The listing builds one solid part. Answer for the finished solid, in the listing's coordinates (mm). Give positions to 0.01 mm unless a question says otherwise; leave off trailing zeros. Loops run counter-clockwise (first coordinate to the right, second up) from the corner with the lowest first, then second, coordinate; pieces in that order, holes last. Notation, with made-up numbers: (81, -39.5) -> (89, -39.5) arc R5 cw to (89, -33.5) -> close; hole circle Ø1 at (-35.75, 65.25). An arc over 180 degrees is marked (long way). One line per question, with ' | ' between items. Start each with the question number.
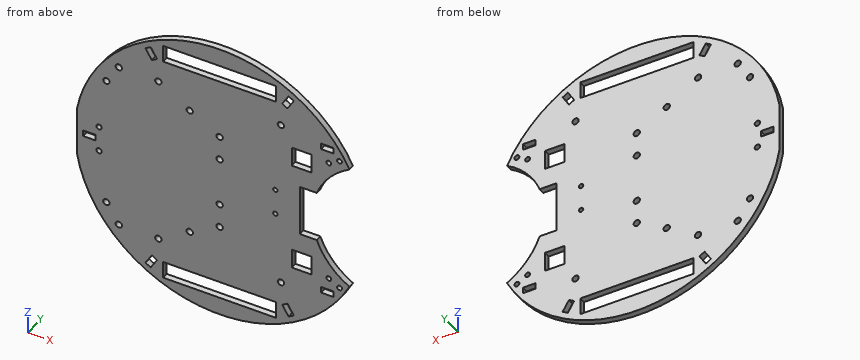
from build123d import *

# Parameters (mm, degrees)
SKETCH1_R           = 1.397
SKETCH1_R_2         = 1.651
SKETCH1_R_3         = 1.143
SKETCH1_R_4         = 1.27
SKETCH1_W           = 58.544107304
SKETCH1_H           = 8.89
SKETCH1_W_2         = 6.35
SKETCH1_H_2         = 3.175
SKETCH1_W_3         = 10.16
SKETCH1_H_3         = 10.16
BOSS_EXTRUDE1_DEPTH = 3.175


with BuildPart() as part:
    # Sketch1 → Boss-Extrude1 (new body)
    with BuildSketch(Plane(origin=(0, 0, 0), x_dir=(1, 0, 0), z_dir=(0, 1, 0))):
        with BuildLine():
            Line((50.342102347, 13.335), (41.582265908, 13.335))
            Line((41.582265908, 13.335), (41.582265908, -13.335))
            Line((41.582265908, -13.335), (50.342102347, -13.335))
            ThreePointArc((50.342102347, -13.335), (52.41895011, -17.937530518), (55.086193863, -22.225))
            ThreePointArc((55.086193863, -22.225), (60.584216496, -28.355013333), (67.270928268, -33.160552015))
            ThreePointArc((67.270928268, -33.160552015), (-10.756431789, -74.224653419), (-73.916912814, -12.7))
            Line((-73.916912814, -12.7), (-73.916912814, 12.7))
            ThreePointArc((-73.916912814, 12.7), (-10.756431789, 74.224653419), (67.270928268, 33.160552015))
            ThreePointArc((67.270928268, 33.160552015), (57.058059725, 24.74076345), (50.342102347, 13.335))
        make_face()
        with Locations(Location((-62.486912814, 6.731, 0), (0, 0, 270))):
            Circle(SKETCH1_R, mode=Mode.SUBTRACT)
        with Locations(Location((-62.486912814, -6.731, 0), (0, 0, 270))):
            Circle(SKETCH1_R, mode=Mode.SUBTRACT)
        with Locations(Location((-31.75, -44.507461806, 0), (0, 0, 270))):
            Circle(SKETCH1_R_2, mode=Mode.SUBTRACT)
        with Locations(Location((31.75, -44.507461806, 0), (0, 0, 270))):
            Circle(SKETCH1_R_2, mode=Mode.SUBTRACT)
        with Locations(Location((31.75, 44.507461806, 0), (0, 0, 90))):
            Circle(SKETCH1_R_2, mode=Mode.SUBTRACT)
        with Locations(Location((0, -12.757461806, 0), (0, 0, 270))):
            Circle(SKETCH1_R_2, mode=Mode.SUBTRACT)
        with Locations(Location((-31.75, 44.507461806, 0), (0, 0, 90))):
            Circle(SKETCH1_R_2, mode=Mode.SUBTRACT)
        with Locations(Location((0, 12.757461806, 0), (0, 0, 90))):
            Circle(SKETCH1_R_2, mode=Mode.SUBTRACT)
        with Locations(Location((28.882265908, 6.731, 0), (0, 0, 270))):
            Circle(SKETCH1_R_3, mode=Mode.SUBTRACT)
        with Locations(Location((-58.676912814, 34.29, 0), (0, 0, 270))):
            Circle(SKETCH1_R_2, mode=Mode.SUBTRACT)
        with Locations(Location((62.141053559, -35.830642926, 0), (0, 0, 270))):
            Circle(SKETCH1_R_4, mode=Mode.SUBTRACT)
        with Locations(Location((56.570777105, -32.679132142, 0), (0, 0, 270))):
            Circle(SKETCH1_R_4, mode=Mode.SUBTRACT)
        with Locations(Location((-58.676912814, -34.29, 0), (0, 0, 270))):
            Circle(SKETCH1_R_2, mode=Mode.SUBTRACT)
        with Locations(Location((28.882265908, -6.731, 0), (0, 0, 270))):
            Circle(SKETCH1_R_3, mode=Mode.SUBTRACT)
        with Locations(Location((0, -25.457461806, 0), (0, 0, 270))):
            Circle(SKETCH1_R_2, mode=Mode.SUBTRACT)
        with Locations(Location((56.570777105, 32.679132142, 0), (0, 0, 90))):
            Circle(SKETCH1_R_4, mode=Mode.SUBTRACT)
        with Locations(Location((62.141053559, 35.830642926, 0), (0, 0, 90))):
            Circle(SKETCH1_R_4, mode=Mode.SUBTRACT)
        with Locations(Location((0, 25.457461806, 0), (0, 0, 90))):
            Circle(SKETCH1_R_2, mode=Mode.SUBTRACT)
        with Locations(Location((-15.496912814, 34.29, 0), (0, 0, 270))):
            Circle(SKETCH1_R_2, mode=Mode.SUBTRACT)
        with Locations(Location((-15.496912814, -34.29, 0), (0, 0, 270))):
            Circle(SKETCH1_R_2, mode=Mode.SUBTRACT)
        with Locations(Location((-52.26766059, -44.507461806, 0), (0, 0, 270))):
            Circle(SKETCH1_R_2, mode=Mode.SUBTRACT)
        with Locations(Location((-52.26766059, 44.507461806, 0), (0, 0, 270))):
            Circle(SKETCH1_R_2, mode=Mode.SUBTRACT)
        with Locations((0, -61.144461806)):
            Rectangle(SKETCH1_W, SKETCH1_H, mode=Mode.SUBTRACT)
        with Locations((0, 61.144461806)):
            Rectangle(SKETCH1_W, SKETCH1_H, mode=Mode.SUBTRACT)
        with Locations((55.791053559, -40.593142926)):
            Rectangle(SKETCH1_W_2, SKETCH1_H_2, mode=Mode.SUBTRACT)
        with Locations((55.791053559, 40.593142926)):
            Rectangle(SKETCH1_W_2, SKETCH1_H_2, mode=Mode.SUBTRACT)
        with Locations((42.456053559, 28.845642926)):
            Rectangle(SKETCH1_W_3, SKETCH1_H_3, mode=Mode.SUBTRACT)
        with Locations((42.456053559, -28.845642926)):
            Rectangle(SKETCH1_W_3, SKETCH1_H_3, mode=Mode.SUBTRACT)
        Polygon((32.44100721, -56.895314679), (35.719111901, -62.333745485), (38.438327304, -60.694693139), (35.160222613, -55.256262334), align=None, mode=Mode.SUBTRACT)
        Polygon((-32.44100721, -56.895314679), (-35.160222613, -55.256262334), (-38.438327304, -60.694693139), (-35.719111901, -62.333745485), align=None, mode=Mode.SUBTRACT)
        Polygon((-35.160222613, 55.256262334), (-38.438327304, 60.694693139), (-35.719111901, 62.333745485), (-32.44100721, 56.895314679), align=None, mode=Mode.SUBTRACT)
        Polygon((35.160222613, 55.256262334), (38.438327304, 60.694693139), (35.719111901, 62.333745485), (32.44100721, 56.895314679), align=None, mode=Mode.SUBTRACT)
        with Locations((-67.566912814, 0)):
            Rectangle(SKETCH1_W_2, SKETCH1_H_2, mode=Mode.SUBTRACT)
    extrude(amount=BOSS_EXTRUDE1_DEPTH)


solid = part.part
1. Straight lines are drawn through the part: L1, parallel to Z at x = -34.5, y = 0.3; L2, parallel to Z at x = -53, y = 2.15; L3, parallel to X at y = 1.4, z = 57.5. For each, find the intervals that lie inside material, in ascending order.
2. Each of these flat-tipped pins is pushed along its axis until it touches: pin 1 Ø1.5 at (x, y) = (45.5, 1.5) entering from +Z; pin 2 Ø1 at (y, z) = (2, -3) entering from +X; pin 3 Ø1.5 at (x, y) = (-49.5, 1.5) entering from -Z. Where does it stop, or does it pass through?
3. The part is cut by section A-A (x = 0). Write down the section's boundary in (y, z) (3 decimals).
4. The part is cut by section D-D (z = 19.5). Write down the section's boundary in (x, y) (3 decimals).
5. The part is cut by section C-C (y = 0.6). Count the separate pieces of the cut face and the enclosed holes in it, plus the area to 3 significant figures.
6. The part is cut by section B-B (x = -21.5). Write down the section's boundary in (y, z) (3 decimals), plus the area to 3 significant figures.
Check sheet entries:
1) L1: z = -66.59 to -60.31, -55.65 to 55.65, 60.31 to 66.59 | L2: z = -53.07 to -45.99, -43.03 to 43.03, 45.99 to 53.07 | L3: x = -48.15 to -36.51, -32.81 to -29.27, 29.27 to 32.81, 36.51 to 48.15
2) pin 1: stops at z = 60.19 | pin 2: stops at x = 41.58 | pin 3: stops at z = -57
3) outline: (0, -75) -> (3.175, -75) -> (3.175, -65.589) -> (0, -65.589) -> close; (0, -56.699) -> (3.175, -56.699) -> (3.175, -27.108) -> (0, -27.108) -> close; (0, -23.806) -> (3.175, -23.806) -> (3.175, -14.408) -> (0, -14.408) -> close; (0, -11.106) -> (3.175, -11.106) -> (3.175, 11.106) -> (0, 11.106) -> close; (0, 14.408) -> (3.175, 14.408) -> (3.175, 23.806) -> (0, 23.806) -> close; (0, 27.108) -> (3.175, 27.108) -> (3.175, 56.699) -> (0, 56.699) -> close; (0, 65.589) -> (3.175, 65.589) -> (3.175, 75) -> (0, 75) -> close
4) outline: (-72.421, 0) -> (53.301, 0) -> (53.301, 3.175) -> (-72.421, 3.175) -> close
5) separate pieces: 1 | enclosed holes: 33 | area: 14,700 mm^2
6) outline: (0, -71.852) -> (3.175, -71.852) -> (3.175, -65.589) -> (0, -65.589) -> close; (0, -56.699) -> (3.175, -56.699) -> (3.175, 56.699) -> (0, 56.699) -> close; (0, 65.589) -> (3.175, 65.589) -> (3.175, 71.852) -> (0, 71.852) -> close | area: 400 mm^2
